For this review, take the finished solid that the model builds, in its own axes (mm). Coordinates: 2 decimals unless noted, no trailing zeros. Write each loop counter-clockwise with the first axis right and the second up, starting at its lowest first coordinate (ties: lowest second). Pieces come first, ordered by that corner, then holes. Notation, with made-up numbers: (-2.75, -19.5) - (24.25, -19.5) arc R30 cw to (24.25, 7.5) - close; hole circle Ø8 at (70.25, 80.5). An arc over 180 degrees is marked (long way). Write each question's results on one line, items separated by ' | '.
Autodesk Inventor part; units mm, degrees
ref_plane "Work Plane1" through (0, 0, 6.16) normal (0, 0, 1) x (1, 0, 0)
ref_plane "Work Plane2" through (0, 0, 2.8) normal (0, 0, 1) x (1, 0, 0)
ref_plane "YZ Plane" through (0, 0, 0) normal (1, 0, 0) x (0, 1, 0)
sketch "Sketch1" plane through (0, 0, 0) normal (0, 0, 1) x (1, 0, 0)
  line L0 (-5.6, 0) -> (5.6, 0) construction
  line L1 (0, -6.4663) -> (0, 6.4663) construction
  line L2 (0, 4.6188) -> (4, 2.3094)
  line L3 (4, 2.3094) -> (4, -2.3094)
  line L4 (4, -2.3094) -> (0, -4.6188)
  line L5 (0, -4.6188) -> (-4, -2.3094)
  line L6 (-4, -2.3094) -> (-4, 2.3094)
  line L7 (-4, 2.3094) -> (0, 4.6188)
  point P0 (0, 0)
  point P1 (0, 0)
  dimension "d67" = 8
extrude "Выдавливание1" add sketch "Sketch1" along normal blind 5.6
ref_plane "Work Plane1" through (0, 0, 6.16) normal (0, 0, 1) x (1, 0, 0)
ref_plane "Work Plane2" through (0, 0, 2.8) normal (0, 0, 1) x (1, 0, 0)
sketch "Sketch2" plane through (0, 0, 5.6) normal (0, 0, 1) x (1, 0, 0)
  point P0 (0, 0)
hole "Отверстие1" at (0, 0, 5.6) direction (0, 0, -1) diameter 4.134 end through all
sketch "Sketch3" plane through (0, 0, 0) normal (1, 0, 0) x (0, 1, 0)
  line L0 (-2.3094, 5.6) -> (2.3094, 5.6) construction
  line L1 (2.3094, 5.6) -> (4.6188, 5.6) construction
  line L2 (-4.6188, 5.6) -> (-2.3094, 5.6) construction
  line L3 (-2.067, 0) -> (-2.067, 5.6) construction
  line L4 (2.3094, 0) -> (2.3094, 5.6) construction
  line L5 (0, -1.12) -> (0, 6.72) construction
  line L6 (-2.5, 5.6) -> (0, 3.1)
  line L7 (0, 3.1) -> (0, 5.6)
  line L8 (0, 5.6) -> (-2.5, 5.6)
  line L9 (2.5, 5.6) -> (0, 3.1)
  line L10 (0, 5.6) -> (2.5, 5.6)
  point P0 (0, 0)
  dimension "d57" = 45
  dimension "d58" = 5
revolve "Вращение1" cut sketch "Sketch3" angle 360 about axis through (0, 0, -10) along (0, 0, 1) contours L8 L7 L6
sketch "Sketch4" plane through (0, 0, 0) normal (1, 0, 0) x (0, 1, 0)
  line L0 (-3.6, 5.6) -> (-6.1, 4.1566)
  line L1 (-6.1, 4.1566) -> (-6.1, 5.6)
  line L2 (0, -1.12) -> (0, 6.72) construction
  line L3 (-3.6, 5.6) -> (-6.1, 5.6)
  line L4 (3.6, 5.6) -> (6.1, 4.1566)
  line L5 (6.1, 4.1566) -> (6.1, 5.6)
  line L6 (3.6, 5.6) -> (6.1, 5.6)
  point P0 (0, 0)
  dimension "d11" = 30
  dimension "d12" = 7.2
  dimension "d13" = 12.2
  dimension "d60" = 5.6
revolve "Вращение2" cut sketch "Sketch4" angle 360 about axis through (0, 0, -10) along (0, 0, 1) contours L0 L1 L3
mirror "ЗеркОтобр1" about plane through (0, 0, 2.8) normal (0, 0, 1) of "Вращение2"
sketch "Sketch5" plane through (0, 0, 0) normal (1, 0, 0) x (0, 1, 0)
  line L0 (2.067, 0) -> (-2.067, 0) construction
  line L1 (0, -1.12) -> (0, 6.72) construction
  line L2 (-2.5, 0) -> (0, 2.5)
  line L3 (0, 0) -> (-2.5, 0)
  line L4 (-2.067, 0) -> (2.067, 0) construction
  line L5 (2.5, 0) -> (-2.5, 0) construction
  line L6 (2.5, 0) -> (0, 2.5)
  line L7 (0, 0) -> (2.5, 0)
  line L8 (0, 2.5) -> (0, 0)
  point P0 (-1.2295, 3.4)
  point P1 (1.2295, 3.4)
  point P2 (-2.067, 5.6)
  dimension "d54" = 45
  dimension "d55" = 5
revolve "Вращение3" cut sketch "Sketch5" angle 360 about axis through (0, 0, -10) along (0, 0, 1) contours L2 L8 L3
equation "\"d67\" = S_"
equation "\"d1\" = m_"
equation "\"d12\" = dw"
equation "\"d13\" = dw + da"
equation "\"d55\" = da"
equation "\"d58\" = da"
equation "\"S_\" = 8"
equation "\"e\" = 8.6"
equation "\"da\" = 5"
equation "\"dw\" = 7.2"
equation "\"m_\" = 5.6"
equation "\"D\" = 5"
equation "\"d15\" = 0.1 * m_"
properties part number "Гайка M5 ГОСТ 15526-70" material "Сталь, мягкая"
Q1. Take a section at B-B on z = 1. State the section outline as (x, y) points.
Results found:
outline: (-4, -2.31) - (0, -4.62) - (4, -2.31) - (4, 2.31) - (0, 4.62) - (-4, 2.31) - close; hole circle Ø4.13 at (0, 0)
Q2. Wall thickness on line 1 along X through (y, z) = (0, 4.25); line 2 along Y through (x, z) = (0.5, 4.65); line 3 along Y through (x, z) = (1.5, 1.85): over which ranges is each line inside the solid? List them lowest first. Write a range as from..to.
Results found:
line 1: -4..-2.07, 2.07..4 | line 2: -4.33..-2.01, 2.01..4.33 | line 3: -3.75..-1.42, 1.42..3.75
Q3. Mouldability with a two-part tool opening along Y and no side actions: class faces 1 (the face through (2.028, -3.448, 2.764)), 2 (the face through (4, 0, 3)), 3 (the face through (-2.028, 3.448, 2.764)), 4 (the face through (1.26, 1.64, 2.77)) as pulls with the +Y half, pulls with the -Y half, needs draft (parallel to the pull), parting line crosses it, or undercut.
Results found:
face 1: pulls with the -Y half | face 2: needs draft | face 3: pulls with the +Y half | face 4: undercut
Q4. For pin 1 (2 mm diameter, centred on x = -1.5, z = 2, fed in from -Y); pin 2 (3 mm diameter, centred on y = 3, z = 4.5, fed in from +X); pin 3 (1.5 mm diameter, centred on x = 2, z = 3, fed in from -Y), all flat-tipped, find the tip position at first contact; note any pin that passes through.
Results found:
pin 1: y = -4.33 | pin 2: x = 4 | pin 3: y = -3.9
Q5. Take a section at A-A on y = 0. State the section outline as (x, z) points, plus the area to 3 significant figures.
Results found:
outline: (-4, 0.23) - (-3.6, 0) - (-2.5, 0) - (-2.07, 0.43) - (-2.07, 5.17) - (-2.5, 5.6) - (-3.6, 5.6) - (-4, 5.37) - close; (2.07, 0.43) - (2.5, 0) - (3.6, 0) - (4, 0.23) - (4, 5.37) - (3.6, 5.6) - (2.5, 5.6) - (2.07, 5.17) - close | area: 21.1 mm2
